Part model, mm, in its own coordinate system. Give positions to 0.01 mm unless a question says otherwise; leave off trailing zeros. Write each loop counter-clockwise with the first axis right and the second up, starting at its lowest first coordinate (ties: lowest second). Pieces come first, ordered by that corner, then holes.
from build123d import *

# Parameters (mm, degrees)
F0_R     = 2.7
F0_R_2   = 2.4
F1_DEPTH = 5
F2_R     = 7.5
F2_R_2   = 2.4
F3_DEPTH = 5
F4_SIZE  = 3
F5_R     = 2


with BuildPart() as f1:
    # F0 (on Top) → F1 (new body)
    with BuildSketch(Plane.XY):
        with BuildLine():
            Line((-10, 20.4), (-10, 0))
            Line((-10, 0), (10, 0))
            Line((10, 0), (10, 20.4))
            ThreePointArc((10, 20.4), (8.424303, 26.599078), (4.079715, 31.293324))
            ThreePointArc((4.079715, 31.293324), (0, 32.5), (-4.079715, 31.293324))
            ThreePointArc((-4.079715, 31.293324), (-8.424303, 26.599078), (-10, 20.4))
        make_face()
        with Locations((0, 10)):
            Circle(F0_R, mode=Mode.SUBTRACT)
        with Locations((0, 25)):
            Circle(F0_R_2, mode=Mode.SUBTRACT)
    extrude(amount=F1_DEPTH)

    # F2 (on face) → F3 (join)
    with BuildSketch(Plane.XY.offset(5)):
        with Locations((0, 25)):
            Circle(F2_R)
        with Locations((0, 25)):
            Circle(F2_R_2, mode=Mode.SUBTRACT)
    extrude(amount=F3_DEPTH)

    # F4
    f4_edges = [f1.edges().sort_by_distance(p)[0] for p in [
        (-7.5, 25, 10),
    ]]
    chamfer(f4_edges, length=F4_SIZE)

    # F5
    f5_edges = [f1.edges().sort_by_distance(p)[0] for p in [
        (-10, 0, 2.5),
        (10, 0, 2.5),
    ]]
    fillet(f5_edges, radius=F5_R)


solid = f1.part
1) Saw through at D-D (x = 1). State how many separate pieces and enclosed holes the cut face has, and give its area (3 significant figures).
Check result:
separate pieces: 3
enclosed holes: 0
area: 159 mm2
2) Saw through at C-C (y = 25). Write the cut outline in (x, z), and give its area (3 significant figures).
Check result:
outline: (-9.16, 0) - (-2.4, 0) - (-2.4, 10) - (-4.5, 10) - (-7.5, 7) - (-7.5, 5) - (-9.16, 5) - close; (2.4, 0) - (9.16, 0) - (9.16, 5) - (7.5, 5) - (7.5, 7) - (4.5, 10) - (2.4, 10) - close
area: 110 mm2
3) Saw through at A-A (y = 10). Write the cut outline in (x, z).
Check result:
outline: (-10, 0) - (-2.7, 0) - (-2.7, 5) - (-10, 5) - close; (2.7, 0) - (10, 0) - (10, 5) - (2.7, 5) - close
4) Mould opens along Y. For faces 1 (the cylindrical face through (-8.38, 26.68, 2.46)), 2 (the cylindrical face through (-0.52, 22.657, 4.93)), 3 (the flat face through (-10, 11, 2)) say: +Y half, -Y half, draft (parallel to the pull), parting line (faces both ways), or undercut.
Check result:
face 1: +Y half
face 2: undercut
face 3: draft
5) Drill centre lines: L1, parallel to Y at x = 0, z = 1.85; L2, parallel to Y at x = 0, z = 6.5; L3, parallel to Z at x = -4.25, y = 8.5. Where is each one in solid material? Low to high.
Check result:
L1: y = 0 to 7.3, 12.7 to 22.6, 27.4 to 32.5
L2: y = 17.5 to 22.6, 27.4 to 32.5
L3: z = 0 to 5
6) Saw through at B-B (z = 9). Write the cut outline in (x, y).
Check result:
outline: circle Ø11 at (0, 25); hole circle Ø4.8 at (0, 25)
